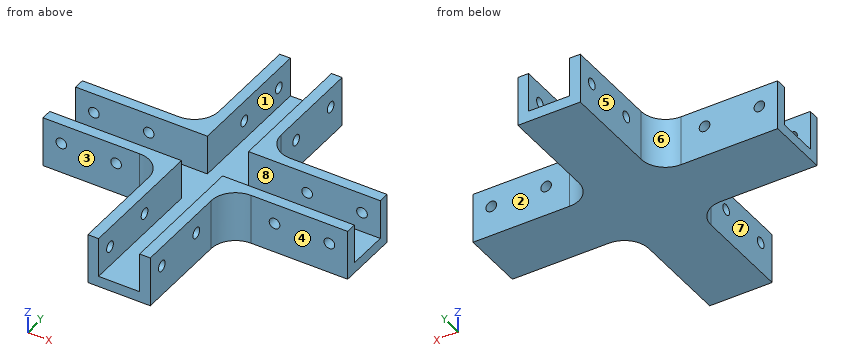
from build123d import *

# Parameters (mm, degrees)
F1_DEPTH = 16.5
F2_W     = 13.5
F2_H     = 13
F3_DEPTH = 100.001
F4_W     = 13.5
F4_H     = 13
F5_DEPTH = 100.001
F6_R     = 1.75
F7_DEPTH = 60.251
F8_R     = 1.75
F9_DEPTH = 60.251
F10_R    = 8


with BuildPart() as f1:
    # F0 (on Top) → F1 (new body)
    with BuildSketch(Plane.XY):
        Polygon((-10.25, 10.25), (-50, 10.25), (-50, -10.25), (-10.25, -10.25), (-10.25, -50), (10.25, -50), (10.25, -10.25), (50, -10.25), (50, 10.25), (10.25, 10.25), (10.25, 50), (-10.25, 50), align=None)
    extrude(amount=F1_DEPTH)

    # F2 (on face) → F3 (cut, through all)
    with BuildSketch(Plane.YZ.offset(50)):
        with Locations((0, 10)):
            Rectangle(F2_W, F2_H)
    extrude(amount=-F3_DEPTH, mode=Mode.SUBTRACT)

    # F4 (on face) → F5 (cut, through all)
    with BuildSketch(Plane.XZ.offset(50)):
        with Locations((0, 10)):
            Rectangle(F4_W, F4_H)
    extrude(amount=-F5_DEPTH, mode=Mode.SUBTRACT)

    # F6 (on face) → F7 (cut, through all)
    with BuildSketch(Plane.YZ.offset(10.25)):
        with Locations((44, 10)):
            Circle(F6_R)
        with Locations((26.000956, 9.814443)):
            Circle(F6_R)
        with Locations((-26.000956, 10.185557)):
            Circle(F6_R)
        with Locations((-44, 10)):
            Circle(F6_R)
    extrude(amount=-F7_DEPTH, mode=Mode.SUBTRACT)

    # F8 (on face) → F9 (cut, through all)
    with BuildSketch(Plane.XZ.offset(10.25)):
        with Locations((44, 10)):
            Circle(F8_R)
        with Locations((26.000956, 9.814443)):
            Circle(F8_R)
        with Locations((-26.000956, 10.185557)):
            Circle(F8_R)
        with Locations((-44, 10)):
            Circle(F8_R)
    extrude(amount=-F9_DEPTH, mode=Mode.SUBTRACT)

    # F10
    f10_edges = [f1.edges().sort_by_distance(p)[0] for p in [
        (10.25, -10.25, 8.25),
        (10.25, 10.25, 8.25),
        (-10.25, 10.25, 8.25),
        (-10.25, -10.25, 8.25),
    ]]
    fillet(f10_edges, radius=F10_R)


solid = f1.part
Design review of the part built by this model. Coordinates are the model's own, in mm. Face numbers are marked on the shaded views. A direction names the side the tool comes from. Round coordinates to 2 decimals unless told otherwise and drop trailing zeros. Order: outer loops, then holes, each group sorted by start corner. A loop starts at its lowest first (then second) coordinate and runs counter-clockwise, first axis right, second up. Notation, with made-up numbers: M 19,-37.5 L 31,-37.5 A19 ccw 31,-24.5 Z; hole C 47,-18 d6. An arc over 180 degrees is marked long. Answer as CSV lines item,"result". Start each with the question number.
1) Add section D-D (x = 37). Give the boundary of the cut face in (y, z).
2) For pin 1 Ø4 at (x, z) = (-26, 10.19) entering from -Y; pin 2 Ø5 at (y, z) = (-28.5, 5) entering from +X; pin 3 Ø5.5 at (y, z) = (-44, 10) entering from -X, all flat-tipped, find the tip position at first contact; note any pin that passes through.
3) The part is to be moulded in two halves that separate along Y. For the marked faces 6, 7 and 8, say which applies: +Y half, -Y half, draft (parallel to the pull), parting line (faces both ways), or undercut.
4) Wall thickness on line 1 along X through (y, z) = (-39, 8.25); line 2 along Z through (x, y) = (44, 9): over which ranges is each line inside the solid? List them lowest first. Write a range as [from, to].
5) Add section A-A (z = 6.25). Give the boundary of the cut face in (x, y), then the cut area to 3 significant figures.
6) Tool access review of the marked faces 1, 2, 3, 4 and 5: name each direction out of +Z, -Z, +X, -X, +Y, -Y from which nothing blocks a thin tool from reaching the whole face with its end or side.
7) Add section B-B (y = 44). Give the boundary of the cut face in (x, z), then the cut area to 3 significant figures.
Resolved:
1,outline,"M -10.25,0 L 10.25,0 L 10.25,16.5 L 6.75,16.5 L 6.75,3.5 L -6.75,3.5 L -6.75,16.5 L -10.25,16.5 Z"
2,pin 1,"y = -10.25"
2,pin 2,"x = 10.25"
2,pin 3,"x = -10.25"
3,face 6,"+Y half"
3,face 7,"draft"
3,face 8,"undercut"
4,line 1,"[-10.25, -6.75], [6.75, 10.25]"
4,line 2,"[0, 8.25], [11.75, 16.5]"
5,outline,"M -50,-10.25 L -18.25,-10.25 A8 cw -10.25,-18.25 L -10.25,-50 L -6.75,-50 L -6.75,-6.75 L -50,-6.75 Z; M -50,6.75 L -6.75,6.75 L -6.75,50 L -10.25,50 L -10.25,18.25 A8 cw -18.25,10.25 L -50,10.25 Z; M 6.75,-50 L 10.25,-50 L 10.25,-18.25 A8 cw 18.25,-10.25 L 50,-10.25 L 50,-6.75 L 6.75,-6.75 Z; M 6.75,6.75 L 50,6.75 L 50,10.25 L 18.25,10.25 A8 cw 10.25,18.25 L 10.25,50 L 6.75,50 Z"
5,area,"1,220 mm^2"
6,face 1,"+Z, +Y, -Y"
6,face 2,"+Z, -Z, +X, +Y"
6,face 3,"+Z, -Z, -X, -Y"
6,face 4,"+Z, -Z, +X, -Y"
6,face 5,"+Z, -Z, -X, +Y"
7,outline,"M -10.25,0 L 10.25,0 L 10.25,8.25 L 6.75,8.25 L 6.75,3.5 L -6.75,3.5 L -6.75,8.25 L -10.25,8.25 Z; M -10.25,11.75 L -6.75,11.75 L -6.75,16.5 L -10.25,16.5 Z; M 6.75,11.75 L 10.25,11.75 L 10.25,16.5 L 6.75,16.5 Z"
7,area,"138 mm^2"
